Here's the drawing with two shaded views (mm, measured from the low corner). I have some questions. Coordinates: 2 decimals unless noted, no trailing zeros. Write each loop counter-clockwise with the first axis right and the second up, starting at its lowest first coordinate (ties: lowest second). Pieces come first, ordered by that corner, then holes.
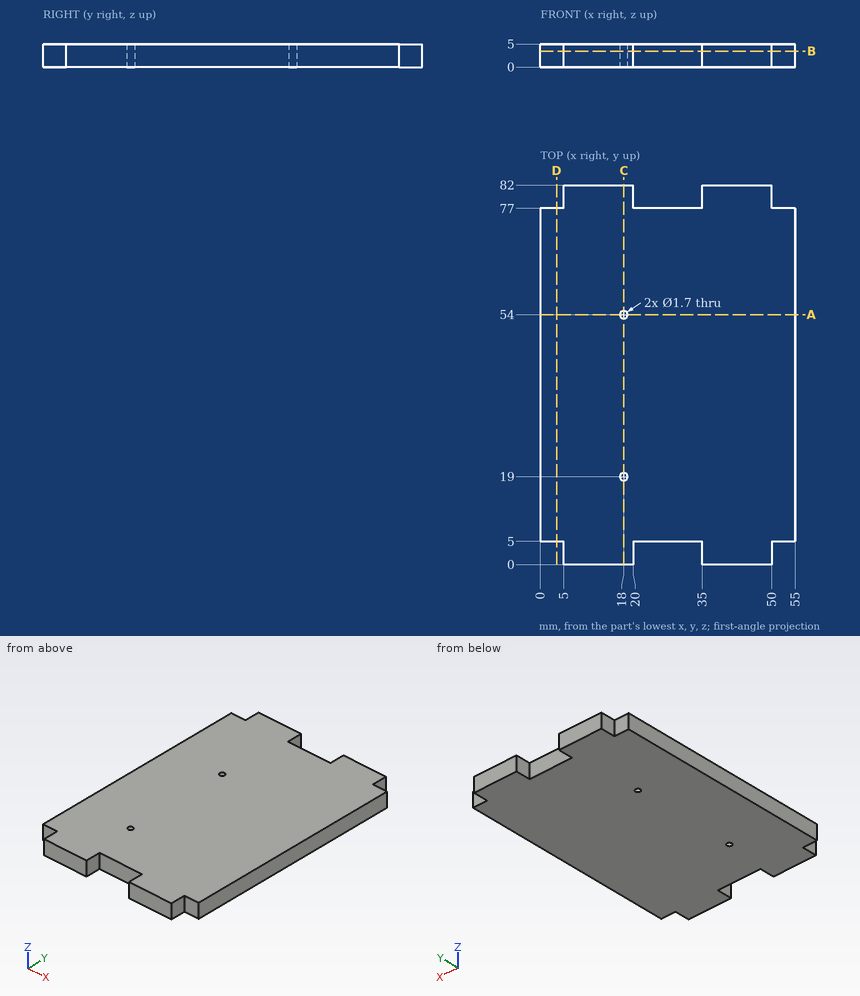
1. If we section it at C-C, the plane x = 18: List the corners of the cut face in (y, z) for me.
2. I'm going to push flat-ended pins straight in: P1, Ø1.5, axis at x = 52.5, z = 1.5, coming from the +Y side; P2, Ø1.5, axis at y = 80.5, z = 2.5, coming from the -X side; P3, Ø2.5, axis at x = 30.5, z = 1.5, coming from the -Y side. Where does each tip first touch, or does it pass through?
3. If I drill on L1, parallel to Y at x = 18, z = 3.95; L2, parallel to X at y = 54, z = 1.7; L3, parallel to Y at x = 4, z = 4.4, over which ranges is the centre line in solid material (lowest first)?
4. If we section it at B-B, the plane z = 3.45: List the corners of the cut face in (x, y) for me, plus the area to 3 significant figures.
5. If we section it at A-A, the plane y = 54: List the corners of the cut face in (x, z) for me, plus the area to 4 significant figures.
6. If we section it at D-D, the plane x = 3.5: List the corners of the cut face in (y, z) for me, plus the area to 3 significant figures.
Answers:
1. outline: (0, 0) - (18.15, 0) - (18.15, 5) - (0, 5) - close; (19.85, 0) - (53.15, 0) - (53.15, 5) - (19.85, 5) - close; (54.85, 0) - (82, 0) - (82, 5) - (54.85, 5) - close
2. P1: stops at y = 77
2. P2: stops at x = 5
2. P3: stops at y = 5
3. L1: y = 0 to 18.15, 19.85 to 53.15, 54.85 to 82
3. L2: x = 0 to 17.15, 18.85 to 55
3. L3: y = 5 to 77
4. outline: (0, 5) - (5, 5) - (5, 0) - (20, 0) - (20, 5) - (35, 5) - (35, 0) - (50, 0) - (50, 5) - (55, 5) - (55, 77) - (50, 77) - (50, 82) - (35, 82) - (35, 77) - (20, 77) - (20, 82) - (5, 82) - (5, 77) - (0, 77) - close; hole circle Ø1.7 at (18, 19); hole circle Ø1.7 at (18, 54)
4. area: 4,260 mm2
5. outline: (0, 0) - (17.15, 0) - (17.15, 5) - (0, 5) - close; (18.85, 0) - (55, 0) - (55, 5) - (18.85, 5) - close
5. area: 266.5 mm2
6. outline: (5, 0) - (77, 0) - (77, 5) - (5, 5) - close
6. area: 360 mm2
